Geometry: final body of the model. Coordinates: model frame, mm. Face numbers are marked on the shaded views. Round coordinates to 2 decimals unless told otherwise and drop trailing zeros. Loops run counter-clockwise (first coordinate to the right, second up) from the corner with the lowest first, then second, coordinate; pieces in that order, holes last. Notation, with made-up numbers: (2.5, 8) -> (54.5, 8) arc R21 cw to (54.5, 28) -> close; hole circle Ø5 at (-7, 7.25). An arc over 180 degrees is marked (long way). Answer in a Markdown table with one row per item.
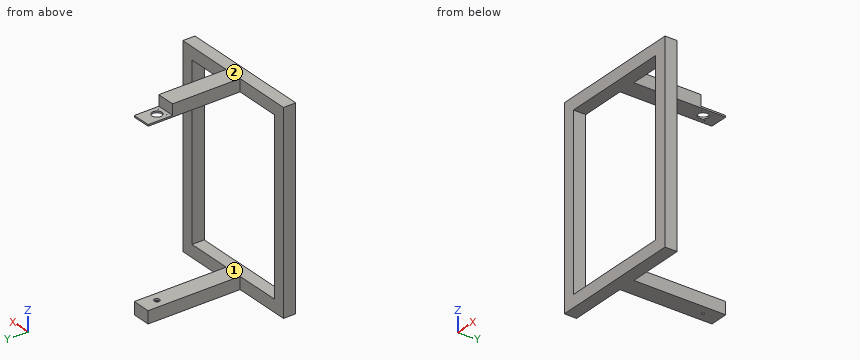
```python
from build123d import *

# Parameters (mm, degrees)
SKETCH1_W           = 454.199999904
SKETCH1_H           = 704.848240034
BOSS_EXTRUDE1_DEPTH = 50.8
SKETCH2_W           = 76.2
SKETCH2_H           = 50.8
BOSS_EXTRUDE2_DEPTH = 279.4
SKETCH4_W           = 76.2
SKETCH4_H           = 50.8
BOSS_EXTRUDE3_DEPTH = 381
SKETCH5_W           = 76.2
SKETCH5_H           = 6.35
BOSS_EXTRUDE4_DEPTH = 101.6
SKETCH6_R           = 1.27
SKETCH6_R_2         = 20.32
CUT_EXTRUDE2_DEPTH  = 6.35
SKETCH8_R           = 11.1125
CUT_EXTRUDE4_DEPTH  = 7.14375
SKETCH9_R           = 5.08
CUT_EXTRUDE5_DEPTH  = 50.8


with BuildPart() as part:
    # Sketch1 → Boss-Extrude1 (new body)
    with BuildSketch(Plane(origin=(0, 0, 0), x_dir=(1, 0, 0), z_dir=(0, 1, 0))):
        Polygon((-277.899999952, 25.4), (277.899999952, 25.4), (277.899999952, -25.4), (277.899999952, -781.048240034), (227.099999952, -781.048240034), (-227.099999952, -781.048240034), (-277.899999952, -781.048240034), (-277.899999952, -25.4), align=None)
        with Locations((0, -377.824120017)):
            Rectangle(SKETCH1_W, SKETCH1_H, mode=Mode.SUBTRACT)
    extrude(amount=BOSS_EXTRUDE1_DEPTH)

    # Sketch2 → Boss-Extrude2 (add)
    with BuildSketch(Plane(origin=(0, 50.8, 0), x_dir=(1, 0, 0), z_dir=(0, 1, 0))):
        with Locations((0, -755.648240034)):
            Rectangle(SKETCH2_W, SKETCH2_H)
    extrude(amount=BOSS_EXTRUDE2_DEPTH)

    # Sketch4 → Boss-Extrude3 (add)
    with BuildSketch(Plane(origin=(0, 50.8, 0), x_dir=(1, 0, 0), z_dir=(0, 1, 0))):
        Rectangle(SKETCH4_W, SKETCH4_H)
    extrude(amount=BOSS_EXTRUDE3_DEPTH)

    # Sketch5 → Boss-Extrude4 (add)
    with BuildSketch(Plane(origin=(0, 330.2, 0), x_dir=(1, 0, 0), z_dir=(0, 1, 0))):
        with Locations((0, -733.423240034)):
            Rectangle(SKETCH5_W, SKETCH5_H)
    extrude(amount=BOSS_EXTRUDE4_DEPTH)

    # Sketch6 → Cut-Extrude2 (cut)
    with BuildSketch(Plane.XY.offset(736.598240034)):
        with Locations((-23.57317231, 390.04634462)):
            Circle(SKETCH6_R)
        with Locations((-23.57317231, 342.9)):
            Circle(SKETCH6_R)
        with Locations((23.57317231, 390.04634462)):
            Circle(SKETCH6_R)
        with Locations((23.57317231, 342.9)):
            Circle(SKETCH6_R)
        with Locations((0, 366.47317231)):
            Circle(SKETCH6_R_2)
    extrude(amount=-CUT_EXTRUDE2_DEPTH, mode=Mode.SUBTRACT)

    # Sketch8 → Cut-Extrude4 (cut)
    with BuildSketch(Plane.XY.offset(25.4)):
        with Locations((0, 366.47317231)):
            Circle(SKETCH8_R)
    extrude(amount=-CUT_EXTRUDE4_DEPTH, mode=Mode.SUBTRACT)

    # Sketch9 → Cut-Extrude5 (cut)
    with BuildSketch(Plane.XY.offset(18.25625)):
        with Locations((0, 366.47317231)):
            Circle(SKETCH9_R)
    extrude(amount=-CUT_EXTRUDE5_DEPTH, mode=Mode.SUBTRACT)


solid = part.part
```
Item 1: Cut plane B-B (y = 222.5). Output: boundary loops of the cut face in (x, z).
Answer:
| item | result |
|---|---|
| outline | (-38.1, -25.4) -> (38.1, -25.4) -> (38.1, 25.4) -> (-38.1, 25.4) -> close; (-38.1, 730.25) -> (38.1, 730.25) -> (38.1, 781.05) -> (-38.1, 781.05) -> close |
Item 2: Draft query along X for the marked faces 1 and 2. Return one class per face: pulls with the +X half, pulls with the -X half, needs draft (parallel to the pull), parting line crosses it, or undercut.
Answer:
| item | result |
|---|---|
| face 1 | undercut |
| face 2 | needs draft |
Item 3: Pin query (flat end, axial travel): pin 1 Ø6.5 at (x, y) = (3.5, 367) entering from +Z; pin 2 Ø3 at (x, y) = (23.57, 390.05) entering from +Z; pin 3 Ø15 at (y, z) = (186.5, 762) entering from -X. Return the tip coordinate at first contact, or that it passes through.
Answer:
| item | result |
|---|---|
| pin 1 | stops at z = 18.26 |
| pin 2 | stops at z = 736.6 |
| pin 3 | stops at x = -38.1 |
Item 4: Line query: probe 1 along X at (y, z) = (342.9, 735); probe 2 along Y at (x, z) = (0, 735); probe 3 along X at (y, z) = (27, 141.5). Output: solid intervals per line, ascending. Write a range as [from, to].
Answer:
| item | result |
|---|---|
| probe 1 | x = [-38.1, -24.84], [-22.3, 22.3], [24.84, 38.1] |
| probe 2 | y = [0, 346.15], [386.79, 431.8] |
| probe 3 | x = [-277.9, -227.1], [227.1, 277.9] |
Item 5: Cut plane A-A (z = 475). Output: boundary loops of the cut face in (x, y), then the cut area to 3 significant figures.
Answer:
| item | result |
|---|---|
| outline | (-277.9, 0) -> (-227.1, 0) -> (-227.1, 50.8) -> (-277.9, 50.8) -> close; (227.1, 0) -> (277.9, 0) -> (277.9, 50.8) -> (227.1, 50.8) -> close |
| area | 5,160 mm² |
